```python
from build123d import *

# Parameters (mm, degrees)
F0_R     = 3.175
F1_DEPTH = 25.4


with BuildPart() as f1:
    # F0 (on Front) → F1 (new body)
    with BuildSketch(Plane.XZ):
        with BuildLine():
            ThreePointArc((44.7334821429, -7.9324362036), (50.1620069047, -5.5115227815), (52.3875, 0))
            ThreePointArc((52.3875, 0), (50.0626600757, 5.6126600757), (44.45, 7.9375))
            ThreePointArc((44.45, 7.9375), (36.5137660501, -0.1417636831), (44.7334821429, -7.9324362036))
        make_face()
        with Locations((44.45, 0)):
            Circle(F0_R, mode=Mode.SUBTRACT)
        with BuildLine():
            ThreePointArc((44.7334821429, -7.9324362036), (36.5137660501, -0.1417636831), (44.45, 7.9375))
            Line((44.45, 7.9375), (18.9322510366, 8.8523612883))
            ThreePointArc((18.9322510366, 8.8523612883), (13.2244578226, 11.5730964697), (11.3073615093, 17.5985462477))
            Line((11.3073615093, 17.5985462477), (15.7942028036, 61.9003804205))
            ThreePointArc((15.7942028036, 61.9003804205), (0, 47.625), (-15.7942028036, 61.9003804205))
            Line((-15.7942028036, 61.9003804205), (-9.525, 0))
            ThreePointArc((-9.525, 0), (0, 9.525), (9.525, 0))
            ThreePointArc((9.525, 0), (6.854408295, -6.6138273281), (0.3401785982, -9.5189234434))
            Line((0.3401785982, -9.5189234434), (44.7334821429, -7.9324362036))
        make_face()
        with BuildLine():
            ThreePointArc((-9.525, 0), (-6.6138273281, -6.854408295), (0.3401785982, -9.5189234434))
            ThreePointArc((0.3401785982, -9.5189234434), (6.854408295, -6.6138273281), (9.525, 0))
            ThreePointArc((9.525, 0), (0, 9.525), (-9.525, 0))
        make_face()
        Circle(F0_R, mode=Mode.SUBTRACT)
        with BuildLine():
            Line((14.9842264132, 68.7429556358), (15.7942028036, 61.9003804205))
            ThreePointArc((15.7942028036, 61.9003804205), (15.8547878338, 62.6991705884), (15.875, 63.5))
            ThreePointArc((15.875, 63.5), (15.6507223365, 66.1590440661), (14.9842264132, 68.7429556358))
        make_face()
        with BuildLine():
            ThreePointArc((-15.7942028036, 61.9003804205), (0, 47.625), (15.7942028036, 61.9003804205))
            Line((15.7942028036, 61.9003804205), (14.9842264132, 68.7429556358))
            ThreePointArc((14.9842264132, 68.7429556358), (0, 79.375), (-14.9842264132, 68.7429556358))
            Line((-14.9842264132, 68.7429556358), (-15.7942028036, 61.9003804205))
        make_face()
        with Locations((0, 63.5)):
            Circle(F0_R, mode=Mode.SUBTRACT)
        with BuildLine():
            ThreePointArc((-14.9842264132, 68.7429556358), (-15.7649337188, 65.3661430393), (-15.7942028036, 61.9003804205))
            Line((-15.7942028036, 61.9003804205), (-14.9842264132, 68.7429556358))
        make_face()
        with BuildLine():
            ThreePointArc((-14.9842264132, 68.7429556358), (0, 79.375), (14.9842264132, 68.7429556358))
            Line((14.9842264132, 68.7429556358), (9.4589602313, 115.4196858236))
            ThreePointArc((9.4589602313, 115.4196858236), (9.5084757244, 114.8608158331), (9.525, 114.3))
            ThreePointArc((9.525, 114.3), (-0.5608158331, 104.7915242756), (-9.4589602313, 115.4196858236))
            Line((-9.4589602313, 115.4196858236), (-14.9842264132, 68.7429556358))
        make_face()
        with Locations((-4.7625, 100.0252)):
            Circle(F0_R, mode=Mode.SUBTRACT)
        with BuildLine():
            ThreePointArc((9.525, 114.3), (9.5084757244, 114.8608158331), (9.4589602313, 115.4196858236))
            ThreePointArc((9.4589602313, 115.4196858236), (0, 123.825), (-9.4589602313, 115.4196858236))
            ThreePointArc((-9.4589602313, 115.4196858236), (-0.5608158331, 104.7915242756), (9.525, 114.3))
        make_face()
        with Locations((0, 114.3)):
            Circle(F0_R, mode=Mode.SUBTRACT)
    extrude(amount=F1_DEPTH)


solid = f1.part
```
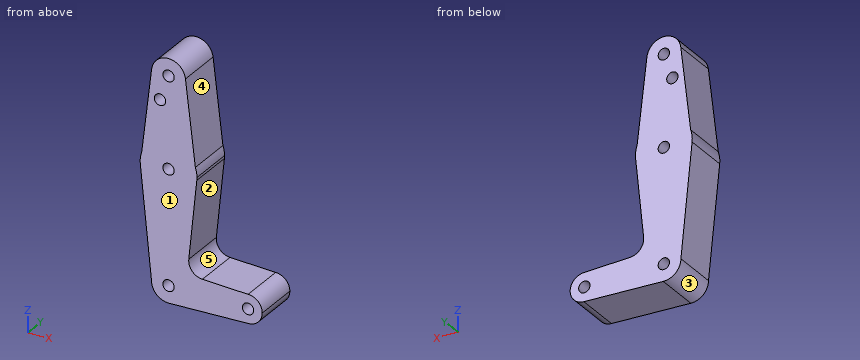
Geometry: final body of the model. Coordinates: model frame, mm. Face numbers are marked on the shaded views. A direction names the side the tool comes from. Coordinates: 2 decimals unless noted, no trailing zeros. Order: outer loops, then holes, each group sorted by start corner. A loop starts at its lowest first (then second) coordinate and runs counter-clockwise, first axis right, second up.
Item 1: Material intervals for line 1 along Z through (x, y) = (44.45, -18) (1 decimal); line 2 along X through (y, z) = (-20.5, 64.5); line 3 along X through (y, z) = (-7, 113.5), sorted ascending.
Answer:
line 1: z = -7.9 to -3.2, 3.2 to 7.9
line 2: x = -15.84 to -3.01, 3.01 to 15.84
line 3: x = -9.69 to -3.07, 3.07 to 9.69
Item 2: Section query A-A (x = 42.5). Output: boundary loops of the cut face in (y, z), then the cut area to 3 significant figures.
Answer:
outline: (-25.4, -8.01) - (0, -8.01) - (0, -2.51) - (-25.4, -2.51) - close; (-25.4, 2.51) - (0, 2.51) - (0, 8.01) - (-25.4, 8.01) - close
area: 280 mm2
Item 3: Contact query for flat-ended pins moving along their axis: P1, Ø8, axis at x = 45, y = -18.5, coming from the -Z side; P2, Ø5.5, axis at x = 0, z = 114.3, coming from the +Y side; P3, Ø2, axis at y = -18.5, z = 74, coming from the -X side; P4, Ø2, axis at x = 6, y = -8, coming from the +Z side. Output: stop coordinate, or through.
Answer:
P1: stops at z = -8.07
P2: passes through
P3: stops at x = -14.48
P4: stops at z = 122.41
Item 4: Section query B-B (y = -10). State how many separate pieces and enclosed holes the cut face has, then the cut area to 3 significant figures.
Answer:
separate pieces: 1
enclosed holes: 5
area: 3,750 mm2
Item 5: Section query D-D (x = 21). Output: boundary loops of the cut face in (y, z).
Answer:
outline: (-25.4, -8.78) - (0, -8.78) - (0, 8.78) - (-25.4, 8.78) - close
Item 6: Draft query along Z for the marked faces 1, 2 and 3. Return one class per face: released by +Z, released by -Z, zero draft, split by the parting line, or undercut.
Answer:
face 1: zero draft
face 2: undercut
face 3: released by -Z
Item 7: Section query C-C (z = 55). Output: boundary loops of the cut face in (x, y).
Answer:
outline: (-15.1, -25.4) - (15.1, -25.4) - (15.1, 0) - (-15.1, 0) - close
Item 8: Access query for the marked faces 4 and 5. Directions: +Z, -Z, +X, -X, +Y, -Y. A direction counts if a zero-diameter tool reaches every point of the face in a straight line with its end or side. Return the directions, or none.
Answer:
face 4: +Z, +X, +Y, -Y
face 5: +X, +Y, -Y
